For this review, take the finished solid that the model builds, in its own axes (mm). Give positions to 0.01 mm unless a question says otherwise; leave off trailing zeros. Write each loop counter-clockwise with the first axis right and the second up, starting at its lowest first coordinate (ties: lowest second). Pieces come first, ordered by that corner, then holes.
1) We need section B-B on z = 1.55. Give the boundary of the cut face in (x, y), and give its area (3 significant figures).
2) Wall thickness on line 1 along X through (y, z) = (-47, 1.7); line 2 along X through (y, z) = (2.5, 1.5); line 3 along Y through (x, z) = (-78, 1.6): over which ranges is each line inside the solid? List them lowest first.
3) We need section C-C on y = 15. Give the boundary of the cut face in (x, z).
4) We need section D-D on x = -58.5. Give the boundary of the cut face in (y, z), and give its area (3 significant figures).
5) We need section A-A on y = -31. Give the boundary of the cut face in (x, z).
from build123d import *

# Parameters (mm, degrees)
SALIENTE_EXTRUIR1_DEPTH = 3


with BuildPart() as part:
    # Croquis1 → Saliente-Extruir1 (new body)
    with BuildSketch(Plane.XY):
        with BuildLine():
            Line((68.287228231, -24.307780687), (68.287228231, -43.400459387))
            Line((68.287228231, -43.400459387), (68.287228231, -53.400459387))
            Line((68.287228231, -53.400459387), (78.287228231, -53.400459387))
            Line((78.287228231, -53.400459387), (78.287228231, 46.599540613))
            Line((78.287228231, 46.599540613), (-89.712771769, 46.599540613))
            Line((-89.712771769, 46.599540613), (-89.712771769, -53.400459387))
            Line((-89.712771769, -53.400459387), (-79.712771769, -53.400459387))
            Line((-79.712771769, -53.400459387), (-79.712771769, -43.400459387))
            Line((-79.712771769, -43.400459387), (-79.712771769, -22.445940721))
            ThreePointArc((-79.712771769, -22.445940721), (-31.962424833, -16.866365463), (0, 19.045062959))
            ThreePointArc((0, 19.045062959), (26.942806363, -13.973710623), (68.287228231, -24.307780687))
        make_face()
    extrude(amount=SALIENTE_EXTRUIR1_DEPTH)


solid = part.part
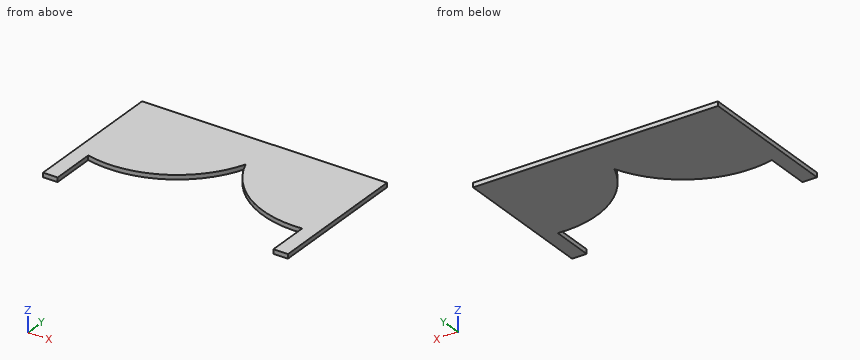
Results list:
1. outline: (-89.71, -53.4) - (-79.71, -53.4) - (-79.71, -22.45) arc R67.59 ccw to (0, 19.05) arc R67.59 ccw to (68.29, -24.31) - (68.29, -53.4) - (78.29, -53.4) - (78.29, 46.6) - (-89.71, 46.6) - close
1. area: 11,000 mm2
2. line 1: x = -89.71 to -79.71, 68.29 to 78.29
2. line 2: x = -89.71 to -9.12, 9.12 to 78.29
2. line 3: y = -22.85 to 46.6
3. outline: (-89.71, 0) - (-1.69, 0) - (-1.69, 3) - (-89.71, 3) - close; (1.69, 0) - (78.29, 0) - (78.29, 3) - (1.69, 3) - close
4. outline: (-24.34, 0) - (46.6, 0) - (46.6, 3) - (-24.34, 3) - close
4. area: 213 mm2
5. outline: (-89.71, 0) - (-79.71, 0) - (-79.71, 3) - (-89.71, 3) - close; (68.29, 0) - (78.29, 0) - (78.29, 3) - (68.29, 3) - close
